Verification items for this drawing (mm, ordinates from the low corner). A direction names the side the tool comes from. Round coordinates to 2 decimals unless told otherwise and drop trailing zeros. Loops run counter-clockwise (first coordinate to the right, second up) from the corner with the lowest first, then second, coordinate; pieces in that order, holes last. Notation, with made-up numbers: M 33,-15.75 L 58,-15.75 A9 cw 58,-4.75 Z; hole C 51,61 d9. An arc over 180 degrees is marked long. One line per item, written item: value.
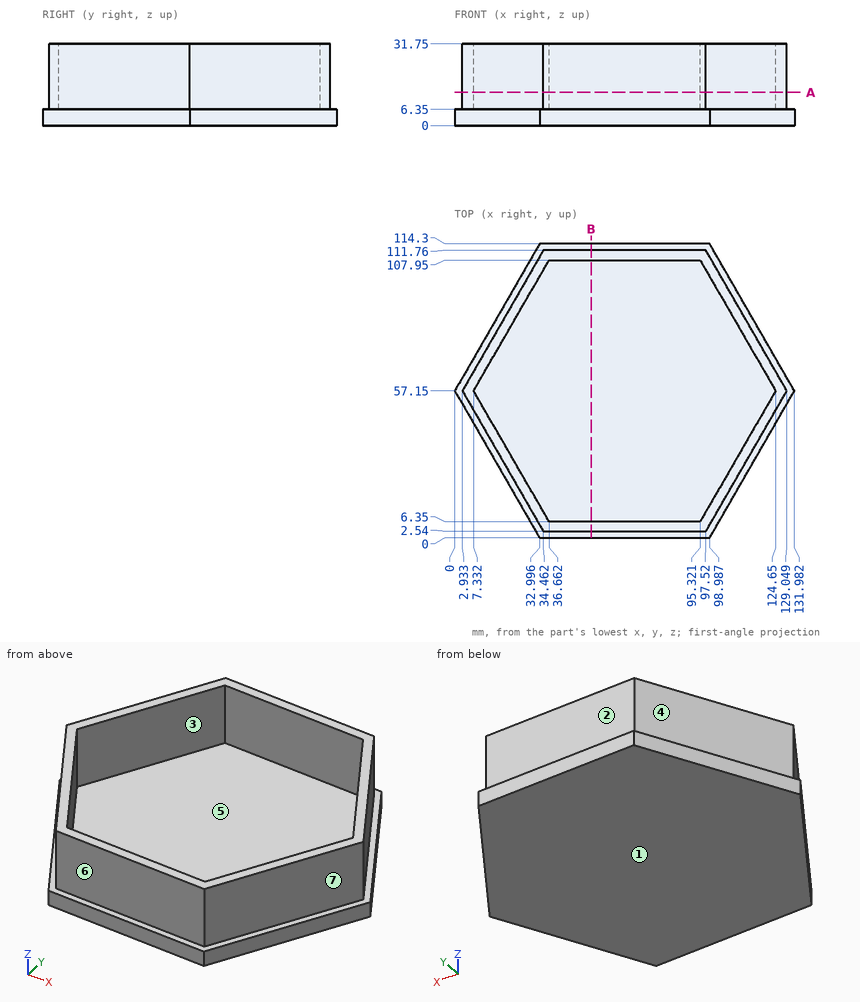
(1) Depth check by flat-ended pin: pin 1 Ø5 at (y, z) = (98, 25) entering from +X; pin 2 Ø2 at (x, z) = (105.5, 25.5) entering from +Y; pin 3 Ø12 at (x, y) = (52.5, 45.5) entering from +Z; pin 4 Ø12 at (x, y) = (93.5, 43.5) entering from -Z. Enter the tip coordinate at first touch or a pass-through.
Completed:
pin 1: stops at x = 106.91
pin 2: stops at y = 99.67
pin 3: stops at z = 6.35
pin 4: stops at z = 0
(2) Sectioned sample at B-B on x = 53. Enter the section's corners in (y, z).
Completed:
outline: M 0,0 L 114.3,0 L 114.3,6.35 L 111.76,6.35 L 111.76,31.75 L 107.95,31.75 L 107.95,6.35 L 6.35,6.35 L 6.35,31.75 L 2.54,31.75 L 2.54,6.35 L 0,6.35 Z
(3) Thickness scan on L1, parallel to Y at x = 54.5, z = 10.5; L2, parallel to Z at x = 73, y = 76; L3, parallel to X at y = 27, z = 7. Record the ranges inside material, lowest first. Write a range as from..to.
Completed:
L1: y = 2.54..6.35, 107.95..111.76
L2: z = 0..6.35
L3: x = 20.34..24.74, 107.24..111.64
(4) Tool access check on the marked faces 1, 2 and 3. Record the directions out of +Z, -Z, +X, -X, +Y, -Y that give a thin tool (end or side, any length) a straight path to the whole face; none if there is none.
Completed:
face 1: -Z, +X, -X, +Y, -Y
face 2: +Z, +X, -X, +Y
face 3: +Z
(5) Mould release check, pull along X, two halves, no side actions. Record for the marked faces 4, 5, 6 and 7: +X half, -X half, draft (parallel to the pull), parting line (faces both ways), or undercut.
Completed:
face 4: -X half
face 5: undercut
face 6: draft
face 7: +X half
(6) Sectioned sample at A-A on z = 13. Enter the section's corners in (x, y).
Completed:
outline: M 2.93,57.15 L 34.46,2.54 L 97.52,2.54 L 129.05,57.15 L 97.52,111.76 L 34.46,111.76 Z; hole M 7.33,57.15 L 36.66,6.35 L 95.32,6.35 L 124.65,57.15 L 95.32,107.95 L 36.66,107.95 Z
